from build123d import *

# Parameters (mm, degrees)
SKETCH1_W               = 10
SKETCH1_H               = 10
BASE_FLANGE1_DEPTH      = 0.7366
EDGE_FLANGE1_DEPTH      = 10
EDGE_FLANGE1_START      = 0.7366
EDGE_FLANGE1_PROFILE_W  = 10
EDGE_FLANGE1_PROFILE_H  = 9.2634
EDGE_FLANGE1_PROFILE_R  = 0.5
EDGE_FLANGE1_FLAT_DEPTH = 0.7366


# Sheet-metal steps are written as plain solids
with BuildPart() as part:
    # Sketch1 → Base-Flange1 (new body)
    with BuildSketch(Plane(origin=(0, 0, 0), x_dir=(1, 0, 0), z_dir=(0, 1, 0))):
        Rectangle(SKETCH1_W, SKETCH1_H)
    extrude(amount=-BASE_FLANGE1_DEPTH)

    # Edge-Flange1 bend section (across the edge) → Edge-Flange1 (add)
    with BuildSketch(Plane(origin=(5.7366, 0, 5), x_dir=(-1, 0, 0), z_dir=(0, 0, -1))):
        with BuildLine():
            Line((-0.7366, 0.7366), (0, 0.7366))
            ThreePointArc((0, 0.7366), (0.215745145, 0.215745145), (0.7366, 0))
            Line((0.7366, 0), (0.7366, -0.7366))
            ThreePointArc((0.7366, -0.7366), (-0.30510971, -0.30510971), (-0.7366, 0.7366))
        make_face()
    extrude(amount=EDGE_FLANGE1_DEPTH)

    # Edge-Flange1 profile (on flange) → Edge-Flange1 flat (add)
    with BuildSketch(Plane(origin=(5.7366, 0, 0), x_dir=(0, 0, -1), z_dir=(1, 0, 0)).offset(EDGE_FLANGE1_START)):
        with Locations((0, 5.3683)):
            Rectangle(EDGE_FLANGE1_PROFILE_W, EDGE_FLANGE1_PROFILE_H)
        with Locations((0, 5)):
            Circle(EDGE_FLANGE1_PROFILE_R, mode=Mode.SUBTRACT)
    extrude(amount=-EDGE_FLANGE1_FLAT_DEPTH)


solid = part.part
Work out the finished part from the listing and answer in its coordinate system (mm). A direction names the side the tool comes from. Coordinates: 2 decimals unless noted, no trailing zeros. Write each loop counter-clockwise with the first axis right and the second up, starting at its lowest first coordinate (ties: lowest second). Pieces come first, ordered by that corner, then holes. Notation, with made-up numbers: M 40,16.25 L 57,16.25 A16 cw 57,29.25 Z; hole C 7,67.5 d9. An arc over 180 degrees is marked long. Write item = value, one per line.
1. The part is cut by section C-C (z = 2.5). Determine the outline of the cut face in (x, y).
Solution:
outline = M -5,-0.74 L 5,-0.74 A1.47 ccw 6.47,0.74 L 6.47,10 L 5.74,10 L 5.74,0.74 A0.74 cw 5,0 L -5,0 Z
2. The part is cut by section D-D (x = -2). Determine the outline of the cut face in (y, z).
Solution:
outline = M -0.74,-5 L 0,-5 L 0,5 L -0.74,5 Z
3. Flat-ended cylindrical pins translate along their axes: pin 1 (5 mm diameter, centred on x = 0, z = 0, fed in from +Y); pin 2 (6 mm diameter, centred on x = 0.5, y = 6, fed in from +Z). Find the tip coordinate at first contact, or state that the pin passes through.
Solution:
pin_1 = 0
pin_2 = through
4. Straight lines are drawn through the part: line 1 (X direction, y = 4.5, z = 2.25); line 2 (Y direction, x = 4, z = -1); line 3 (Y direction, x = 6.05, z = 0). For each, find the intervals that lie inside material, in ascending order. Write a range as from..to.
Solution:
line_1 = 5.74..6.47
line_2 = -0.74..0
line_3 = -0.3..4.5, 5.5..10
5. The part is cut by section B-B (z = 0). Determine the outline of the cut face in (x, y).
Solution:
outline = M -5,-0.74 L 5,-0.74 A1.47 ccw 6.47,0.74 L 6.47,4.5 L 5.74,4.5 L 5.74,0.74 A0.74 cw 5,0 L -5,0 Z; M 5.74,5.5 L 6.47,5.5 L 6.47,10 L 5.74,10 Z
6. For faces 4 (the face through (0, -0.737, 0)), 5 (the face through (5.737, 4, 0)), determine the directions among +Z, -Z, +X, -X, +Y, -Y from which every point of the face is accessible in a straight line to the end or side of a thin tool.
Solution:
face_4 = +Z, -Z, +X, -X, -Y
face_5 = +Z, -Z, -X, +Y
7. Determine the mould class of faces 1 (the face through (0, 0, 0)), 2 (the face through (3.3, -0.2, 5)), 3 (the face through (6.11, 5.496, 0.065)) for opening direction Y: released by +Y, released by -Y, zero draft, split by the parting line, or undercut.
Solution:
face_1 = released by +Y
face_2 = zero draft
face_3 = undercut
8. The part is cut by section A-A (y = 5). Determine the outline of the cut face in (x, z), then the cut area to 3 significant figures.
Solution:
outline = M 5.74,-5 L 6.47,-5 L 6.47,-0.5 L 5.74,-0.5 Z; M 5.74,0.5 L 6.47,0.5 L 6.47,5 L 5.74,5 Z
area = 6.63 mm2
